```python
from build123d import *

# Parameters (mm, degrees)
SKETCH1_W           = 28
SKETCH1_H           = 35
SKETCH1_R           = 1.625
BOSS_EXTRUDE1_DEPTH = 6.35
BOSS_EXTRUDE2_DEPTH = 35
SKETCH3_W           = 6
SKETCH3_H           = 6.5
SKETCH3_W_2         = 15
SKETCH3_H_2         = 6
SKETCH3_R           = 1.25
CUT_EXTRUDE1_DEPTH  = 6.35
SKETCH4_W           = 27
SKETCH4_H           = 26.166174209
CUT_EXTRUDE2_DEPTH  = 3.175
FILLET1_R           = 2
FILLET2_R           = 6.35
FILLET3_R           = 2


with BuildPart() as part:
    # Sketch1 → Boss-Extrude1 (new body)
    with BuildSketch(Plane(origin=(0, 0, 0), x_dir=(1, 0, 0), z_dir=(0, 1, 0))):
        Rectangle(SKETCH1_W, SKETCH1_H)
        with Locations(Location((4, 7.5, 0), (0, 0, 270))):
            Circle(SKETCH1_R, mode=Mode.SUBTRACT)
        with Locations(Location((4, -7.5, 0), (0, 0, 270))):
            Circle(SKETCH1_R, mode=Mode.SUBTRACT)
    extrude(amount=BOSS_EXTRUDE1_DEPTH)

    # Sketch2 → Boss-Extrude2 (add)
    with BuildSketch(Plane.XY.offset(17.5)):
        Polygon((-14, 0), (-30.833087105, 29.155762114), (-25.333825791, 32.330762114), (-10.333825791, 6.35), align=None)
    extrude(amount=-BOSS_EXTRUDE2_DEPTH)

    # Sketch3 → Cut-Extrude1 (cut)
    with BuildSketch(Plane(origin=(-10.5, -6.062177826, 0), x_dir=(0, 0, 1), z_dir=(-0.8660254037844415, -0.4999999999999949, 0))):
        with Locations((-10.5, 28.416174209)):
            Rectangle(SKETCH3_W, SKETCH3_H)
        with Locations((0, 28.416174209)):
            Rectangle(SKETCH3_W_2, SKETCH3_H)
        with Locations((0, 34.666174209)):
            Rectangle(SKETCH3_W_2, SKETCH3_H_2)
        with Locations(Location((-10.5, 34.666174209, 0), (0, 0, 270))):
            Circle(SKETCH3_R)
        with Locations(Location((-10.5, 22.166174209, 0), (0, 0, 270))):
            Circle(SKETCH3_R)
        with Locations(Location((10.5, 22.166174209, 0), (0, 0, 270))):
            Circle(SKETCH3_R)
        with Locations(Location((10.5, 34.666174209, 0), (0, 0, 270))):
            Circle(SKETCH3_R)
        with Locations((10.5, 28.416174209)):
            Rectangle(SKETCH3_W, SKETCH3_H)
        with Locations((0, 22.166174209)):
            Rectangle(SKETCH3_W_2, SKETCH3_H_2)
    extrude(amount=-CUT_EXTRUDE1_DEPTH, mode=Mode.SUBTRACT)

    # Sketch4 → Cut-Extrude2 (cut)
    with BuildSketch(Plane(origin=(-10.5, -6.062177826, 0), x_dir=(0, 0, 1), z_dir=(-0.8660254037844417, -0.49999999999999484, 0))):
        with Locations((0, 6.083087105)):
            Rectangle(SKETCH4_W, SKETCH4_H)
    extrude(amount=-CUT_EXTRUDE2_DEPTH, mode=Mode.SUBTRACT)

    # Fillet1
    fillet1_edges = [part.edges().sort_by_distance(p)[0] for p in [
        (-18.708271776, 11.329965932, 7.5),
        (-18.708271776, 11.329965932, 13.5),
        (-18.708271776, 11.329965932, -13.5),
        (-20.333456448, 17.319868355, -7.5),
        (-20.333456448, 17.319868355, -13.5),
        (-23.583456448, 22.949033479, -13.5),
        (-23.583456448, 22.949033479, -7.5),
        (-26.583456448, 28.145185902, -7.5),
        (-26.583456448, 28.145185902, 7.5),
        (-23.583456448, 22.949033479, 7.5),
        (-23.583456448, 22.949033479, 13.5),
        (-20.333456448, 17.319868355, 13.5),
        (-20.333456448, 17.319868355, 7.5),
        (-18.708271776, 11.329965932, -7.5),
    ]]
    fillet(fillet1_edges, radius=FILLET1_R)

    # Fillet2
    fillet2_edges = [part.edges().sort_by_distance(p)[0] for p in [
        (-14, 0, 15.5),
        (-14, 0, -15.5),
        (-10.333825791, 6.35, 0),
        (-28.083456448, 30.743262114, 17.5),
        (-28.083456448, 30.743262114, -17.5),
        (-10.333825791, 0, 0),
    ]]
    fillet(fillet2_edges, radius=FILLET2_R)

    # Fillet3
    fillet3_edges = [part.edges().sort_by_distance(p)[0] for p in [
        (-15.958641119, 12.917465932, 7.5),
        (-15.958641119, 12.917465932, -7.5),
    ]]
    fillet(fillet3_edges, radius=FILLET3_R)


solid = part.part
```
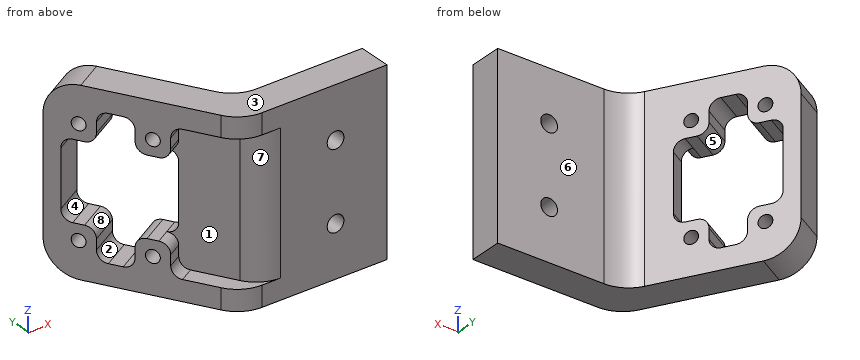
CAD build for the part. Positions are in the model's coordinates, mm. Face numbers are marked on the shaded views. A direction names the side the tool comes from. Give positions to 0.01 mm unless a question says otherwise; leave off trailing zeros. Loops run counter-clockwise (first coordinate to the right, second up) from the corner with the lowest first, then second, coordinate; pieces in that order, holes last. Notation, with made-up numbers: M 70,-17 L 121,-17 A25 cw 121,10 Z; hole C 2.25,8 d4. An arc over 180 degrees is marked long. Use one line per item in the form item = value.
Item 1: Slice it at C-C (x = -14). List the corners of the cut face in (y, z).
Determined:
outline = M 1.17,-17.5 L 12.7,-17.5 L 12.7,17.5 L 1.17,17.5 L 1.17,13.5 L 6.35,13.5 L 6.35,-13.5 L 1.17,-13.5 Z
Item 2: Which spindle directions (+Z, -Z, +X, -X, +Y, -Y) get a long thin tool onto all of the face, cutting with end or side? Do the marked faces 4, 5, 6, 7 and 8. Say none if no direction does.
Determined:
face_4 = +X, -Y
face_5 = -X
face_6 = +Z, -Z, +X, +Y
face_7 = -X, -Y
face_8 = +X
Item 3: Flat gauge pins, fed straight in: pin 1 (5 mm diameter, centred on x = 4, z = -7.5, fed in from +Y); pin 2 (10 mm diameter, centred on x = 4, y = 14.5, fed in from +Z); pin 3 (4 mm diameter, centred on y = 27, z = -10, fed in from -X); pin 4 (6 mm diameter, centred on y = 25.5, z = 2.5, fed in from -X). Where does each tip first touch, or does it go through?
Determined:
pin_1 = 6.35
pin_2 = through
pin_3 = -30.74
pin_4 = -30.45
Item 4: Two-plate mould, pull along Y, no slides. Class the marked faces 1, 2 and 3: pulls with the +Y half, pulls with the -Y half, needs draft (parallel to the pull), parting line crosses it, or undercut.
Determined:
face_1 = pulls with the -Y half
face_2 = undercut
face_3 = needs draft
Item 5: Slice it at B-B (x = 4). List the corners of the cut face in (y, z) (3 decimals), plus the area to 3 significant figures.
Determined:
outline = M 0,-17.5 L 6.35,-17.5 L 6.35,-9.125 L 0,-9.125 Z; M 0,-5.875 L 6.35,-5.875 L 6.35,5.875 L 0,5.875 Z; M 0,9.125 L 6.35,9.125 L 6.35,17.5 L 0,17.5 Z
area = 181 mm2
Item 6: Drill centre lines: probe 1 along Y at (x, z) = (4.5, 5.5); probe 2 along X at (y, z) = (2.25, 7.5) (3 decimals); probe 3 along X at (y, z) = (4.25, -7.5) (3 decimals). Where is each one in solid material? Low to high. Write a range as from..to.
Determined:
probe_1 = 0..6.35
probe_2 = -11.517..2.375, 5.625..14
probe_3 = -12.788..2.375, 5.625..14
Item 7: Slice it at A-A (z = -3). List the corners of the cut face in (x, y) (3 decimals).
Determined:
outline = M -30.833,29.156 L -29.333,26.558 L -23.834,29.733 L -25.334,32.331 Z; M -17.333,12.124 L -12.167,3.175 A6.35 ccw -6.668,0 L 14,0 L 14,6.35 L -6.668,6.35 A6.35 cw -12.167,9.525 L -14.584,13.711 Z
Item 8: Slice it at D-D (z = 15). List the corners of the cut face in (x, y) (3 decimals), plus the area to 3 significant figures.
Determined:
outline = M -30.183,28.03 L -15.833,3.175 A6.35 ccw -10.334,0 L 14,0 L 14,6.35 L -6.668,6.35 A6.35 cw -12.167,9.525 L -24.684,31.205 Z
area = 360 mm2
